Geometry: final body of the model. Coordinates: model frame, mm. A direction names the side the tool comes from. Round coordinates to 2 decimals unless told otherwise and drop trailing zeros. Loops run counter-clockwise (first coordinate to the right, second up) from the corner with the lowest first, then second, coordinate; pieces in that order, holes last. Notation, with made-up numbers: (86.5, 14) - (115.5, 14) arc R9 cw to (115.5, 20) - close; hole circle Ø3 at (10, -2). An arc over 180 degrees is marked (long way). Use CSV: the item, a comma, the result in double quotes.
Autodesk Inventor part; units mm, degrees
ref_plane "YZ Plane" through (0, 0, 0) normal (1, 0, 0) x (0, 1, 0)
ref_plane "XZ Plane" through (0, 0, 0) normal (0, 1, 0) x (-1, 0, 0)
ref_plane "XY Plane" through (0, 0, 0) normal (0, 0, 1) x (1, 0, 0)
sketch "스케치1" plane through (0, 0, 0) normal (0, 0, 1) x (1, 0, 0)
  line L0 (38.7711, -20.2424) -> (-38.7711, -20.2424)
  line L1 (-38.7711, -20.2424) -> (-38.7711, 20.2424)
  line L2 (-38.7711, 20.2424) -> (38.7711, 20.2424)
  line L3 (38.7711, 20.2424) -> (38.7711, -20.2424)
  line L4 (38.7711, -20.2424) -> (-38.7711, 20.2424) construction
  line L5 (-38.7711, -20.2424) -> (38.7711, 20.2424) construction
  point P0 (0, 0)
extrude "돌출1" add sketch "스케치1" along normal blind 40
sketch "스케치2" plane through (0, 0, 40) normal (0, 0, 1) x (1, 0, 0)
  line L0 (38.7711, 20.2424) -> (-38.7711, 20.2424)
  line L1 (-30.6833, 20.2424) -> (-30.6833, -13.1037)
  line L2 (-30.6833, -13.1037) -> (-22.1205, -13.1037)
  line L3 (38.7711, -20.2424) -> (38.7711, 20.2424)
  line L4 (38.7711, -13.1037) -> (22.0956, -13.1037)
  arc A0 (22.0956, -13.1037) -> (-22.1205, -13.1037) centre (-0.0125, -25.2018) ccw
  line L5 (-30.6833, 20.2424) -> (38.7711, 20.2424)
  line L6 (38.7711, -13.1037) -> (38.7711, 20.2424)
  circle A1 centre (-0.0125, -25.2018) radius 17.0581
  point P0 (0, 0)
extrude "돌출2" cut sketch "스케치2" against normal blind 40
sketch "스케치3" plane through (-38.7711, -20.2424, 0) normal (0, -1, 0) x (1, 0, 0)
  circle A0 centre (38.7711, 19.9954) radius 2.1048
  point P0 (38.7711, 0)
extrude "돌출3" cut sketch "스케치3" against normal blind 30.75
sketch "스케치4" plane through (22.0956, -13.1037, 40) normal (0, 1, 0) x (1, 0, 0)
  circle A0 centre (7.6344, 28.4237) radius 4
  circle A1 centre (7.6344, 8.2529) radius 4
  point P0 (-22.0956, 40)
  dimension "d7" = 8
  dimension "d8" = 8
extrude "돌출4" cut sketch "스케치4" against normal blind 30.75
sketch "스케치5" plane through (-30.6833, -13.1037, 40) normal (1, 0, 0) x (0, 0, -1)
  line L0 (16, 33.3461) -> (16, 22.7148)
  line L1 (0, 33.3461) -> (40, 33.3461)
  line L2 (24, 33.3461) -> (24, 19.5161)
  line L3 (40, 33.3461) -> (40, 0)
  line L4 (0, 0) -> (0, 33.3461)
  arc A0 (16, 19.5161) -> (24, 19.5161) centre (20, 19.5161) ccw
  line L5 (16, 33.3461) -> (24, 33.3461)
  line L6 (16, 19.5161) -> (16, 22.7148)
  point P0 (40, 13.1037)
  dimension "d11" = 16
  dimension "d12" = 16
extrude "돌출5" cut sketch "스케치5" against normal blind 30.75
fillet "모깎기1" radius 5 4 edges at (-34.7272, 20.2424, 40) (-34.7272, 20.2424, 0) (38.7711, -16.673, 40) (38.7711, -16.673, 0)
properties part number "240628_final3"
Item 1: Reachability of faces 4 (the cylindrical face through (37.345, -16.723, 38.496)), 5 (the flat face through (-35, 13, 24)), 6 (the flat face through (-30.683, 0, 20)) from +Z, -Z, +X, -X, +Y, -Y: full face, straight path, thin tool, end or side. Return the list, or none.
Final values:
face 4,"+Z, +X, +Y, -Y"
face 5,"+X, -X, +Y"
face 6,"+Z, -Z, +Y"
Item 2: Section D-D on z = 34. Return the cut outline in (x, y), plus the area to 3 significant figures.
Final values:
outline,"(-38.77, -20.24) - (-16.33, -20.24) arc R17.06 cw to (16.31, -20.24) - (26.42, -20.24) - (26.42, -13.1) - (22.1, -13.1) arc R25.2 ccw to (-22.12, -13.1) - (-30.68, -13.1) - (-30.68, 20.24) - (-38.77, 20.24) - close; (33.04, -20.24) - (38.77, -20.24) - (38.77, -13.1) - (33.04, -13.1) - close"
area,"898 mm²"
Item 3: Section C-C on z = 6. Return the cut outline in (x, y), plus the area to 3 significant figures.
Final values:
outline,"(-38.77, -20.24) - (-16.33, -20.24) arc R17.06 cw to (16.31, -20.24) - (38.77, -20.24) - (38.77, -13.1) - (22.1, -13.1) arc R25.2 ccw to (-22.12, -13.1) - (-30.68, -13.1) - (-30.68, 20.24) - (-38.77, 20.24) - close"
area,"945 mm²"
Item 4: Mould query, pull axis X, two halves, no side actions, for faces 1 (the cylindrical face through (-34.671, 2.413, 20.088)), 2 (the flat face through (38.771, -17, 20)), 3 (the cylindrical face through (0, 0, 16)). Classes: released by +X, released by -X, zero draft, split by the parting line, or undercut.
Final values:
face 1,"zero draft"
face 2,"released by +X"
face 3,"undercut"
Item 5: Section A-A on x = 29.73. Return the cut outline in (y, z), plus the area to 3 significant figures.
Final values:
outline,"(-20.24, 0) - (-13.1, 0) - (-13.1, 7.58) - (-20.24, 7.58) - close; (-20.24, 15.58) - (-13.1, 15.58) - (-13.1, 27.75) - (-20.24, 27.75) - close; (-20.24, 35.75) - (-13.1, 35.75) - (-13.1, 40) - (-20.24, 40) - close"
area,"171 mm²"
Item 6: Pin query (flat end, axial travel): P1, Ø1.5, axis at x = -18.5, z = 17.5, coming from the +Y side; P2, Ø5, axis at x = 5, z = 20.5, coming from the -Y side; P3, Ø4.5, axis at x = -27.5, z = 10, coming from the +Y side. Return the tip coordinate at first contact, or that it passes through.
Final values:
P1,"stops at y = -7.3"
P2,"stops at y = -9.89"
P3,"stops at y = -13.1"
Item 7: Section B-B on x = 0. Return the cut outline in (y, z).
Final values:
outline,"(-8.14, 0) - (0, 0) - (0, 17.89) - (-8.14, 17.89) - close; (-8.14, 22.1) - (0, 22.1) - (0, 40) - (-8.14, 40) - close"
Item 8: Material intervals for line 1 (Z direction, x = 29.73, y = -18.75); line 2 (Z direction, x = 29, y = -16); line 3 (Z direction, x = 0, y = -4), sorted ascending.
Final values:
line 1,"z = 0 to 7.58, 15.58 to 27.75, 35.75 to 40"
line 2,"z = 0 to 7.64, 15.51 to 27.81, 35.68 to 40"
line 3,"z = 0 to 17.89, 22.1 to 40"
